Input: part model. Units: mm. Frame: model coordinates. Face numbers are marked on the shaded views. A direction names the side the tool comes from. Coordinates: 2 decimals unless noted, no trailing zeros. Loops run counter-clockwise (first coordinate to the right, second up) from the corner with the lowest first, then second, coordinate; pieces in that order, holes last.
Item 1: Section D-D on x = -82. Return loops of the section in (y, z).
Item 2: Section C-C on z = -7. Return loops of the section in (x, y), and give its area (3 significant figures).
Item 3: Ray query, line 1 along X through (y, z) = (-25, 17); line 2 along Z through (x, y) = (17.5, -35); line 3 along X through (y, z) = (-3, -2). Return the intervals inside material, ascending.
Item 4: Section B-B on y = -43.5. Return loops of the section in (x, z), and give its area (3 significant figures).
Item 5: Section A-A on x = -46.5. Return loops of the section in (y, z), and give its area (3 significant figures).
Item 6: Contact query for flat-ended pins moving along their axis: P1, Ø10, axis at x = -56, z = 16.5, coming from the +Y side; P2, Ø6, axis at x = -50.5, y = -21.5, coming from the -Z side; P3, Ø1.5, axis at x = -43, z = 19, coming from the -Y side; P4, Ø1.5, axis at x = -40, z = 32.5, coming from the +Y side. Output: stop coordinate, or through.
Item 7: Reachability of the marked faces 1, 2 and 3 from +Z, -Z, +X, -X, +Y, -Y: full face, straight path, thin tool, end or side. Return the list, or none.
```python
from build123d import *

# Parameters (mm, degrees)
F1_DEPTH = 50.8
F2_R     = 2.073956
F2_R_2   = 2.230105
F3_DEPTH = 25.4
F4_DEPTH = 52.51404
F5_R     = 2.54
F6_DEPTH = 7.10246


with BuildPart() as f1:
    # F0 (on Front) → F1 (new body)
    with BuildSketch(Plane.XZ):
        with BuildLine():
            ThreePointArc((-33.760353, 38.253132), (-38.232387, 36.383421), (-40.08238, 31.903194))
            Line((-40.08238, 31.903194), (-40.08238, -16.708975))
            ThreePointArc((-40.08238, -16.708975), (-38.222508, -21.199103), (-33.73238, -23.058975))
            Line((-33.73238, -23.058975), (23.82785, -23.058975))
            ThreePointArc((23.82785, -23.058975), (28.317978, -21.199103), (30.17785, -16.708975))
            Line((30.17785, -16.708975), (30.17785, 32.156763))
            ThreePointArc((30.17785, 32.156763), (28.308077, 36.65677), (23.799877, 38.506701))
            Line((23.799877, 38.506701), (-33.760353, 38.253132))
        make_face()
    extrude(amount=F1_DEPTH)

    # F2 (on face) → F3 (join)
    with BuildSketch(Plane(origin=(-40.08238, 0, 0), x_dir=(0, -1, 0), z_dir=(-1, 0, 0))):
        Polygon((14.87593, 25.757497), (9.62919, 21.33056), (14.87593, 15.591938), (35.209692, 15.591938), (41.109629, 21.33056), (35.209692, 25.757497), align=None)
        with Locations((18.483063, 21.33056)):
            Circle(F2_R, mode=Mode.SUBTRACT)
        with Locations((31.599913, 21.33056)):
            Circle(F2_R_2, mode=Mode.SUBTRACT)
    extrude(amount=F3_DEPTH)

    # F2 (on face) → F4 (join)
    with BuildSketch(Plane(origin=(-40.08238, 0, 0), x_dir=(0, -1, 0), z_dir=(-1, 0, 0))):
        with Locations((18.483063, 21.33056)):
            Circle(F2_R)
        with Locations((31.599913, 21.33056)):
            Circle(F2_R_2)
    extrude(amount=F4_DEPTH)

    # F5 (on face) → F6 (cut)
    with BuildSketch(Plane.YZ.offset(30.17785)):
        with Locations((-27.174922, 14.381909)):
            Circle(F5_R)
    extrude(amount=-F6_DEPTH, mode=Mode.SUBTRACT)


solid = f1.part
```
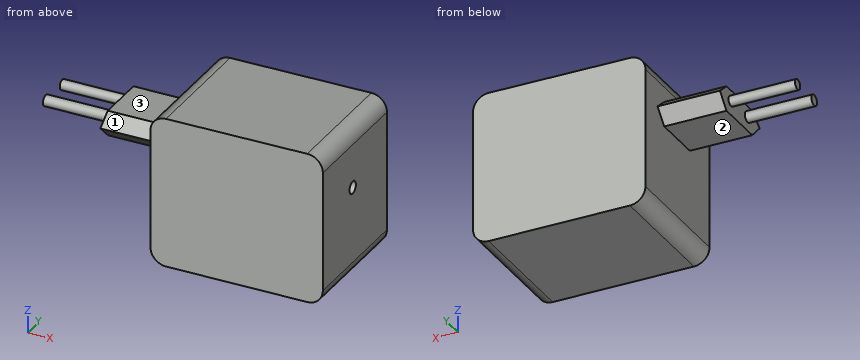
Results found:
1. outline: circle Ø4.46 at (-31.6, 21.33); circle Ø4.15 at (-18.48, 21.33)
2. outline: (-40.08, -50.8) - (30.18, -50.8) - (30.18, 0) - (-40.08, 0) - close
2. area: 3,570 mm2
3. line 1: x = -65.48 to 30.18
3. line 2: z = -23.06 to 38.48
3. line 3: x = -40.08 to 30.18
4. outline: (-40.08, -16.71) arc R6.35 ccw to (-33.73, -23.06) - (23.83, -23.06) arc R6.35 ccw to (30.18, -16.71) - (30.18, 32.16) arc R6.35 ccw to (23.8, 38.51) - (-33.76, 38.25) arc R6.35 ccw to (-40.08, 31.9) - close
4. area: 4,280 mm2
5. outline: (-41.11, 21.33) - (-35.21, 15.59) - (-14.88, 15.59) - (-9.63, 21.33) - (-14.88, 25.76) - (-35.21, 25.76) - close
5. area: 263 mm2
6. P1: stops at y = -9.63
6. P2: stops at z = 15.59
6. P3: stops at y = -39.48
6. P4: stops at y = 0
7. face 1: +Z, -X, -Y
7. face 2: -Z, -X, +Y, -Y
7. face 3: +Z, -X, +Y, -Y
